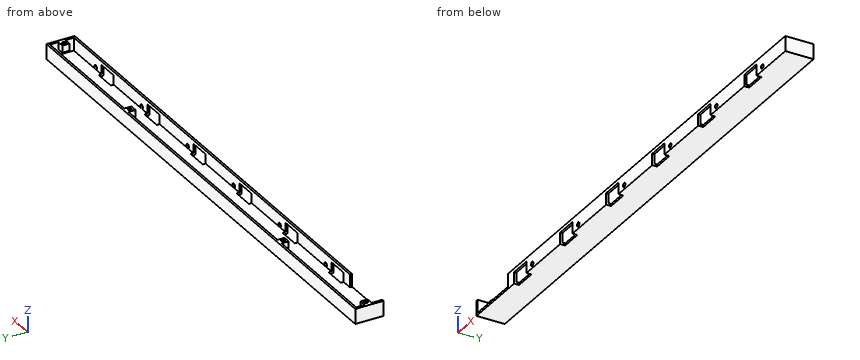
Autodesk Inventor part; units mm, degrees
ref_plane "YZ Plane" through (0, 0, 0) normal (1, 0, 0) x (0, 1, 0)
ref_plane "XZ Plane" through (0, 0, 0) normal (0, 1, 0) x (-1, 0, 0)
ref_plane "XY Plane" through (0, 0, 0) normal (0, 0, 1) x (1, 0, 0)
sketch "Skizze1" plane through (0, 0, 0) normal (0, 0, 1) x (1, 0, 0)
  line L0 (-188.78, 10) -> (188.78, 10)
  line L1 (188.78, 10) -> (188.78, -10)
  line L2 (188.78, -10) -> (-188.78, -10)
  line L3 (-188.78, -10) -> (-188.78, 10)
  line L4 (-264.292, 0) -> (264.292, 0) construction
  line L5 (0, -14) -> (0, 14) construction
  point P0 (0, 0)
  dimension "d0" = 377.56
  dimension "d1" = 20
extrude "Extrusion1" add sketch "Skizze1" along normal blind 10.6
sketch "Skizze2" plane through (0, 0, 10.6) normal (0, 0, 1) x (1, 0, 0)
  line L0 (-187.28, 8.5) -> (187.28, 8.5)
  line L1 (187.28, 8.5) -> (187.28, -8.5)
  line L2 (187.28, -8.5) -> (-187.28, -8.5)
  line L3 (-187.28, -8.5) -> (-187.28, 8.5)
  line L4 (-264.292, 0) -> (264.292, 0) construction
  line L5 (0, -14) -> (0, 14) construction
  line L6 (-188.78, -10) -> (188.78, -10) construction
  line L7 (188.78, -10) -> (188.78, 10) construction
  point P0 (0, 0)
  dimension "d4" = 1.5
  dimension "d5" = 1.5
extrude "Extrusion2" cut sketch "Skizze2" against normal blind 9.1
sketch "Skizze3" plane through (-188.78, -10, 0) normal (0, -1, 0) x (1, 0, 0)
  line L0 (0, 0) -> (377.56, 0)
  line L1 (377.56, 0) -> (377.56, 10.6)
  line L2 (0, 10.6) -> (377.56, 10.6)
  line L3 (0, 0) -> (0, 10.6)
  point P0 (188.78, 0)
  point P1 (349.43, 3)
  dimension "d9" = 28.13
  dimension "d10" = 3
hole "Bohrung1" at (160.65, -10, 3) direction (0, 1, 0) diameter 3 depth 1.5
pattern_linear "Rechteckige Anordnung1" count 6 spacing 56.26 along (-1, 0, 0) of "Bohrung1"
sketch "Skizze4" plane through (-188.78, -10, 0) normal (0, -1, 0) x (1, 0, 0)
  circle A0 centre (68.13, 3) radius 1.5
  circle A1 centre (124.39, 3) radius 1.5
  circle A2 centre (180.65, 3) radius 1.5
  circle A3 centre (236.91, 3) radius 1.5
  circle A4 centre (293.17, 3) radius 1.5
  circle A5 centre (349.43, 3) radius 1.5
  line L0 (0, 0) -> (377.56, 0)
  line L1 (377.56, 0) -> (377.56, 10.6)
  line L2 (0, 10.6) -> (377.56, 10.6)
  line L3 (0, 0) -> (0, 10.6)
  line L4 (38.5, 10.6) -> (38.5, 0) construction
  line L5 (1.5, 10.6) -> (1.5, 1.5)
  line L6 (38.5, 1.5) -> (1.5, 1.5)
  line L7 (1.5, 1.5) -> (1.5, 10.6)
  line L8 (1.5, 10.6) -> (38.5, 10.6)
  line L9 (38.5, 10.6) -> (38.5, 1.5)
  point P0 (188.78, 0)
  dimension "d21" = 29.63
extrude "Extrusion3" cut sketch "Skizze4" against normal up to surface (1.5 mm away) contours L2 L9 L6 L5
sketch "Skizze5" plane through (-188.78, -10, 0) normal (0, -1, 0) x (1, 0, 0)
  line L0 (0, 0) -> (377.56, 0)
  line L1 (342.43, 0) -> (327.43, 0)
  line L2 (327.43, 0) -> (327.43, 8.1)
  line L3 (327.43, 8.1) -> (342.43, 8.1)
  line L4 (342.43, 8.1) -> (342.43, 0)
  line L5 (38.5, 10.6) -> (377.56, 10.6)
  line L6 (377.56, 0) -> (377.56, 10.6)
  circle A0 centre (349.43, 3) radius 1.5
  point P0 (188.78, 0)
  point P1 (327.43, 0)
  dimension "d24" = 15
  dimension "d25" = 2.5
  dimension "d27" = 7
extrude "Extrusion4" cut sketch "Skizze5" against normal blind 3.5 contours L2 L3 L4 L0
pattern_linear "Rechteckige Anordnung2" count 6 spacing 56.26 along (-1, 0, 0) of "Extrusion4"
sketch "Skizze7" plane through (0, 0, 10.6) normal (0, 0, 1) x (1, 0, 0)
  line L0 (-187.28, -10) -> (-187.28, 8.5)
  line L1 (-187.28, -2.5) -> (-182.28, -2.5)
  line L2 (-182.28, -2.5) -> (-182.28, 2.5)
  line L3 (-182.28, 2.5) -> (-187.28, 2.5)
  line L4 (-187.28, 2.5) -> (-187.28, -2.5)
  line L5 (-264.292, 0) -> (264.292, 0) construction
  line L6 (0, -14) -> (0, 14)
  line L7 (-187.28, 8.5) -> (187.28, 8.5)
  line L8 (-96.14, 8.5) -> (-91.14, 8.5)
  line L9 (-91.14, 8.5) -> (-91.14, 3.5)
  line L10 (-91.14, 3.5) -> (-96.14, 3.5)
  line L11 (-96.14, 3.5) -> (-96.14, 8.5)
  circle A0 centre (-184.78, 0) radius 1.25
  circle A1 centre (-93.64, 6) radius 1.25
  point P0 (0, 0)
  dimension "d36" = 5
  dimension "d37" = 5
  dimension "d38" = 5
  dimension "d39" = 5
  dimension "d40" = 91.14
  dimension "d41" = 91.14
  dimension "d42" = 2.5
  dimension "d43" = 2.5
  dimension "d44" = 93.64
  dimension "d45" = 6
  dimension "d46" = 184.78
extrude "Extrusion6" add sketch "Skizze7" against normal blind 5
mirror "Spiegeln2" about plane through (0, 0, 0) normal (1, 0, 0) of "Extrusion6"
properties part number "PCB_Kabelkanal_1.0"
Geometry check sheet. Reference: the model listing, model coordinates, mm. Coordinates: 2 decimals unless noted, no trailing zeros. Loops run counter-clockwise (first coordinate to the right, second up) from the corner with the lowest first, then second, coordinate; pieces in that order, holes last. Notation, with made-up numbers: (44.5, -28) - (64.5, -28) arc R6 cw to (64.5, -21) - close; hole circle Ø11 at (80, 16). An arc over 180 degrees is marked (long way). Use one line per item in the form item = value. Start each with the question number.
Item 1: Section check A-A, the plane x = -162.5. Enter the section's corners in (y, z), and give its area (4 significant figures).
Item 2: Thickness scan on probe 1 along Y at (x, z) = (-184.78, 7.4); probe 2 along Y at (x, z) = (-93.64, 9.5); probe 3 along Y at (x, z) = (184.78, 6.7). Record the ranges inside material, lowest first.
Item 3: Gauge pin test, flat ends, axial feed: pin 1 (0.8 mm diameter, centred on x = 31.5, y = -9, fed in from -Z); pin 2 (1.5 mm diameter, centred on x = -7.5, y = 7.5, fed in from +Z); pin 3 (0.8 mm diameter, centred on x = -79, z = 0.5, fed in from -Y). Record the tip position at first contact, or that the pin passes through.
Computed:
q1.outline = (-10, 0) - (10, 0) - (10, 10.6) - (8.5, 10.6) - (8.5, 1.5) - (-10, 1.5) - close
q1.area = 43.65 mm2
q2.probe_1 = -2.5 to -1.25, 1.25 to 2.5, 8.5 to 10
q2.probe_2 = -10 to -8.5, 3.5 to 4.75, 7.25 to 10
q2.probe_3 = -10 to -8.5, -2.5 to -1.25, 1.25 to 2.5, 8.5 to 10
q3.pin_1 = 8.1
q3.pin_2 = 1.5
q3.pin_3 = -6.5
